from build123d import *

# Parameters (mm, degrees)
BOSS_EXTRUDE1_DEPTH      = 15
BOSS_EXTRUDE1_DEPTH_BACK = 30
SKETCH2_R                = 5
CUT_EXTRUDE1_DEPTH       = 53.966825438


with BuildPart() as part:
    # Sketch1 → Boss-Extrude1 (new, two sides: drawn at the far end of the back side and taken through both)
    with BuildSketch(Plane(origin=(0, 0, 0), x_dir=(1, 0, 0), z_dir=(0, 1, 0)).offset(-BOSS_EXTRUDE1_DEPTH_BACK)):
        with BuildLine():
            ThreePointArc((15, -33.275366264), (-9.757930329, -35.171477019), (-30, -20.790622886))
            Line((-30, -20.790622886), (-30, -52.5))
            Line((-30, -52.5), (15, -52.5))
            Line((15, -52.5), (15, -33.275366264))
        make_face()
    extrude(amount=BOSS_EXTRUDE1_DEPTH + BOSS_EXTRUDE1_DEPTH_BACK)

    # Sketch2 → Cut-Extrude1 (cut, through all)
    with BuildSketch(Plane.XY.offset(52.5)):
        with Locations((0, -20)):
            Circle(SKETCH2_R)
        with Locations((0, 5)):
            Circle(SKETCH2_R)
    extrude(amount=-CUT_EXTRUDE1_DEPTH, mode=Mode.SUBTRACT)


solid = part.part
Can you work these out from the model? Positions are in its coordinate system, mm. Give positions to 0.01 mm unless a question says otherwise; leave off trailing zeros. Loops run counter-clockwise (first coordinate to the right, second up) from the corner with the lowest first, then second, coordinate; pieces in that order, holes last. Notation, with made-up numbers: M 56.25,-29.75 L 115.25,-29.75 A15 ccw 115.25,-20.75 Z; hole C 6,47 d8. An arc over 180 degrees is marked long. One line per item, written item: value. Start each with the question number.
1) Thinking about a two-plate mould opening in X: for faces 1 (the face through (-30, -8, 36)), 2 (the face through (15, -8, 43)), 3 (the face through (-8, -30, 43)), 4 (the face through (-9.416, -7.815, 35.265)), which applies, +X half, -X half, draft (parallel to the pull), parting line (faces both ways), or undercut?
2) If we section it at C-C, the plane y = 5: Write out the boundary of the cut face in (x, z).
3) If we section it at D-D, the plane y = -3: Write out the boundary of the cut face in (x, z), and give its area (3 significant figures).
4) If we section it at B-B, the plane z = 41.5: Write out the boundary of the cut face in (x, y), and give its area (3 significant figures).
5) I'm going to push flat-ended pins straight in: pin 1 (9 mm diameter, centred on x = 0, y = -20, fed in from +Z); pin 2 (1.5 mm diameter, centred on x = 3, y = -7, fed in from -Z); pin 3 (2 mm diameter, centred on y = -23.5, z = 26, fed in from +X). Where does each tip first touch, or does it pass through?
6) If we section it at A-A, the plane x = 0: Write out the boundary of the cut face in (y, z).
7) If I drill on line 1 (Y direction, x = 0, z = 46); line 2 (X direction, y = 5, z = 45); line 3 (X direction, y = 2, z = 38), over which ranges is the centre line in solid material (lowest first)? Write a range as [from, to].
Completed:
1. face 1: -X half
1. face 2: +X half
1. face 3: draft
1. face 4: undercut
2. outline: M -30,20.79 A36.5 cw -5,36.16 L -5,52.5 L -30,52.5 Z; M 5,36.16 A36.5 cw 15,33.28 L 15,52.5 L 5,52.5 Z
3. outline: M -30,20.79 A36.5 cw 15,33.28 L 15,52.5 L -30,52.5 Z
3. area: 876 mm^2
4. outline: M -30,-30 L 15,-30 L 15,15 L -30,15 Z; hole C 0,-20 d10; hole C 0,5 d10
4. area: 1,870 mm^2
5. pin 1: passes through
5. pin 2: stops at z = 36.31
5. pin 3: stops at x = -24.56
6. outline: M -30,36.5 L -25,36.5 L -25,52.5 L -30,52.5 Z; M -15,36.5 L 0,36.5 L 0,52.5 L -15,52.5 Z; M 10,36.5 L 15,36.5 L 15,52.5 L 10,52.5 Z
7. line 1: y = [-30, -25], [-15, 0], [10, 15]
7. line 2: x = [-30, -5], [5, 15]
7. line 3: x = [-30, -4], [4, 15]
